Can you work these out from the model? Positions are in its coordinate system, mm. A direction names the side the tool comes from. Coordinates: 2 decimals unless noted, no trailing zeros. Write each loop counter-clockwise with the first axis right and the second up, starting at its lowest first coordinate (ties: lowest second). Pieces come first, ordered by that corner, then holes. Notation, with made-up numbers: (11.25, 30.5) - (42.25, 30.5) arc R24 ccw to (42.25, 61.5) - close; hole circle Ø5 at (54.5, 89.5). An arc over 180 degrees is marked (long way). One line per question, with ' | ' between items. Start each with the question number.
from build123d import *

# Parameters (mm, degrees)
SKETCH1_W           = 47
SKETCH1_H           = 24
SKETCH1_W_2         = 44
SKETCH1_H_2         = 21
BOSS_EXTRUDE1_DEPTH = 1
SKETCH1_3_W         = 47
SKETCH1_3_H         = 24
SKETCH1_3_W_2       = 44
SKETCH1_3_H_2       = 21
BOSS_EXTRUDE2_DEPTH = 10
SKETCH2_W           = 1.5
SKETCH2_H           = 2.861016429
SKETCH2_H_2         = 2.980642968
SKETCH2_H_3         = 2.463825615
SKETCH2_H_4         = 2.315157892
CUT_EXTRUDE1_DEPTH  = 9


with BuildPart() as part:
    # Sketch1 → Boss-Extrude1 (new body)
    with BuildSketch(Plane(origin=(0, 0, 0), x_dir=(1, 0, 0), z_dir=(0, 1, 0))):
        Rectangle(SKETCH1_W, SKETCH1_H)
        Rectangle(SKETCH1_W_2, SKETCH1_H_2, mode=Mode.SUBTRACT)
        Rectangle(SKETCH1_W_2, SKETCH1_H_2)
    extrude(amount=BOSS_EXTRUDE1_DEPTH)

    # Sketch1<3> → Boss-Extrude2 (add)
    with BuildSketch(Plane(origin=(0, 0, 0), x_dir=(1, 0, 0), z_dir=(0, 1, 0))):
        Rectangle(SKETCH1_3_W, SKETCH1_3_H)
        Rectangle(SKETCH1_3_W_2, SKETCH1_3_H_2, mode=Mode.SUBTRACT)
    extrude(amount=BOSS_EXTRUDE2_DEPTH)

    # Sketch2 → Cut-Extrude1 (cut)
    with BuildSketch(Plane(origin=(0, 10, 0), x_dir=(1, 0, 0), z_dir=(0, 1, 0))):
        with Locations((22.75, 9.069491786)):
            Rectangle(SKETCH2_W, SKETCH2_H)
        with Locations((22.75, -9.009678516)):
            Rectangle(SKETCH2_W, SKETCH2_H_2)
        with Locations((-22.75, 9.268087193)):
            Rectangle(SKETCH2_W, SKETCH2_H_3)
        with Locations((-22.75, -9.342421054)):
            Rectangle(SKETCH2_W, SKETCH2_H_4)
    extrude(amount=-CUT_EXTRUDE1_DEPTH, mode=Mode.SUBTRACT)


solid = part.part
(1) I'm going to push flat-ended pins straight in: pin 1 (1.5 mm diameter, centred on y = 3, z = 9, fed in from -X); pin 2 (8 mm diameter, centred on x = -15, z = 0, fed in from +Y). Where does each tip first touch, or does it pass through?
(2) If we section it at A-A on y = 2.75: List the corners of the cut face in (x, z) for me.
(3) If we section it at B-B on x = -20.5: List the corners of the cut face in (y, z) for me.
(4) If we section it at C-C on z = -5.5: List the corners of the cut face in (x, y) for me, plus the area to 3 significant figures.
(5) If I drill on probe 1 along Z at (x, y) = (5, 6.75); probe 2 along X at (y, z) = (2.75, -5.5); probe 3 along Y at (x, z) = (-1.5, -9.25), over which ranges is the centre line in solid material (lowest first)?
(6) If we mould it in two halves opening along Z, with no side actions, what happens to faces 4 (the face through (0, 5, -12)), 5 (the face through (-23, 10, 0)), 6 (the face through (22, 5, 0))? For each: +Z half, -Z half, draft (parallel to the pull), parting line (faces both ways), or undercut.
(7) Which directions (+Z, -Z, +X, -X, +Y, -Y) give clear straight access to the entire face, cutting with the end or side of a thin tool? Please do faces 1 (the face through (23, 6, 7.519)), 2 (the face through (-23, 6, 8.185)), 3 (the face through (-22, 5, 0)).
Values:
1) pin 1: through | pin 2: y = 1
2) outline: (-23.5, -12) - (23.5, -12) - (23.5, -10.5) - (-23.5, -10.5) - close; (-23.5, -8.04) - (-22, -8.04) - (-22, 8.18) - (-23.5, 8.18) - close; (-23.5, 10.5) - (23.5, 10.5) - (23.5, 12) - (-23.5, 12) - close; (22, -7.64) - (23.5, -7.64) - (23.5, 7.52) - (22, 7.52) - close
3) outline: (0, -12) - (10, -12) - (10, -10.5) - (1, -10.5) - (1, 10.5) - (10, 10.5) - (10, 12) - (0, 12) - close
4) outline: (-23.5, 0) - (23.5, 0) - (23.5, 10) - (22, 10) - (22, 1) - (-22, 1) - (-22, 10) - (-23.5, 10) - close | area: 74.0 mm2
5) probe 1: -12 to -10.5, 10.5 to 12 | probe 2: -23.5 to -22, 22 to 23.5 | probe 3: 0 to 1
6) face 4: -Z half | face 5: draft | face 6: undercut
7) face 1: +X, +Y | face 2: +X, -X, +Y | face 3: +Y
